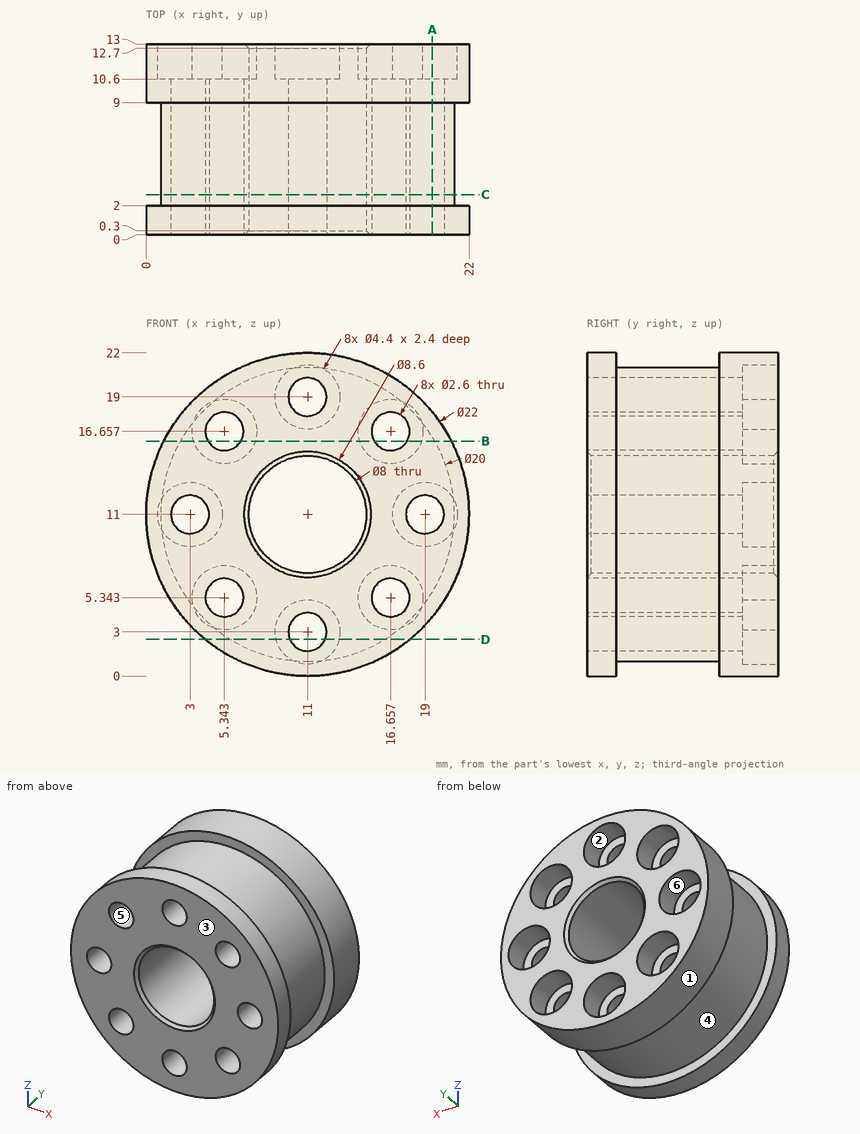
Geometry check sheet. Reference: drawing and pictorial views, mm from the part's lowest x, y, z. A direction names the side the tool comes from. Coordinates: 2 decimals unless noted, no trailing zeros. Order: outer loops, then holes, each group sorted by start corner. A loop starts at its lowest first (then second) coordinate and runs counter-clockwise, first axis right, second up. Notation, with made-up numbers: (33.25, -26.5) - (43.25, -26.5) arc R29 cw to (43.25, 12.5) - close; hole circle Ø4 at (-38, 48). An arc over 180 degrees is marked (long way). Answer in a Markdown table with one row per item. Add a question column.
1) Material ranges on line 1 along X through (y, z) = (12.1, 11); line 2 along X through (y, z) = (7, 17.5), recorded low to high. Write a range as [from, to].
2) Cross-section at C-C, the plane y = 2.75. State how many separate pieces and enclosed holes the cut face has, then the cut area to 3 significant figures.
3) Cross-section at D-D, the plane z = 2.5. Record the cut outline in (x, y), then the cut area to 3 significant figures.
4) Gauge pin test, flat ends, axial feed: P1, Ø4, axis at x = 17.5, z = 6.5, coming from the -Y side; P2, Ø1.3, axis at x = 6, z = 4.5, coming from the +Y side; P3, Ø5, axis at x = 4, y = 5, coming from the -Z side; P4, Ø6, axis at y = 10.5, z = 3, coming from the +X side. Record the tip position at first contact, or that the pin passes through.
5) Cross-section at A-A, the plane x = 19.5. Record the cut outline in (y, z), then the cut area to 3 significant figures.
6) Cross-section at B-B, the plane z = 16. Record the cut outline in (x, y) (1 decimal), then the cut area to 3 significant figures.
7) Set-up check for the marked faces 4, 5 and 6: record each of +Z, -Z, +X, -X, +Y, -Y from which the full face is reachable in a straight line by a thin tool's end or side.
8) Release check for a two-part mould opening along X. For the marked faces 1, 2 and 3 record: +X half, -X half, draft (parallel to the pull), parting line (faces both ways), or undercut.
Check result:
| question | item | result |
|---|---|---|
| 1 | line 1 | x = [0, 0.8], [5.2, 7], [15, 16.8], [21.2, 22] |
| 1 | line 2 | x = [3.4, 4.35], [6.33, 15.67], [17.65, 18.6] |
| 2 | separate pieces | 1 |
| 2 | enclosed holes | 9 |
| 2 | area | 221 mm² |
| 3 | outline | (4.02, 0) - (9.8, 0) - (9.8, 10.6) - (8.86, 10.6) - (8.86, 13) - (4.02, 13) - (4.02, 9) - (5.73, 9) - (5.73, 2) - (4.02, 2) - close; (12.2, 0) - (17.98, 0) - (17.98, 2) - (16.27, 2) - (16.27, 9) - (17.98, 9) - (17.98, 13) - (13.14, 13) - (13.14, 10.6) - (12.2, 10.6) - close |
| 3 | area | 122 mm² |
| 4 | P1 | stops at y = 0 |
| 4 | P2 | stops at y = 10.6 |
| 4 | P3 | stops at z = 2.07 |
| 4 | P4 | stops at x = 20.8 |
| 5 | outline | (0, 4.02) - (2, 4.02) - (2, 5.73) - (9, 5.73) - (9, 4.02) - (13, 4.02) - (13, 8.86) - (10.6, 8.86) - (10.6, 9.8) - (0, 9.8) - close; (0, 12.2) - (10.6, 12.2) - (10.6, 13.14) - (13, 13.14) - (13, 17.98) - (9, 17.98) - (9, 16.27) - (2, 16.27) - (2, 17.98) - (0, 17.98) - close |
| 5 | area | 122 mm² |
| 6 | outline | (1.2, 0) - (4.2, 0) - (4.2, 10.6) - (3.2, 10.6) - (3.2, 13) - (1.2, 13) - (1.2, 9) - (2.3, 9) - (2.3, 2) - (1.2, 2) - close; (6.5, 0) - (15.5, 0) - (15.5, 10.6) - (14.6, 10.6) - (14.6, 13) - (7.4, 13) - (7.4, 10.6) - (6.5, 10.6) - close; (17.8, 0) - (20.8, 0) - (20.8, 2) - (19.7, 2) - (19.7, 9) - (20.8, 9) - (20.8, 13) - (18.8, 13) - (18.8, 10.6) - (17.8, 10.6) - close |
| 6 | area | 171 mm² |
| 7 | face 4 | none |
| 7 | face 5 | +Y, -Y |
| 7 | face 6 | +Y |
| 8 | face 1 | parting line |
| 8 | face 2 | undercut |
| 8 | face 3 | draft |
